Autodesk Inventor part; units mm, degrees
ref_plane "YZ Plane" through (0, 0, 0) normal (1, 0, 0) x (0, 1, 0)
ref_plane "XZ Plane" through (0, 0, 0) normal (0, 1, 0) x (-1, 0, 0)
ref_plane "XY Plane" through (0, 0, 0) normal (0, 0, 1) x (1, 0, 0)
sketch "Sketch1" plane through (0, 0, 0) normal (0, 0, 1) x (1, 0, 0)
  circle A0 centre (0, 0) radius 2.5
  dimension "d0" = 5
extrude "Extrusion1" add sketch "Sketch1" along normal blind 105
sketch "Sketch2" plane through (0, 0, 105) normal (0, 0, 1) x (1, 0, 0)
  circle A0 centre (0, 0) radius 2.5
  circle A1 centre (0, 0) radius 2.5
  circle A2 centre (0, 0) radius 3.75
  dimension "d3" = 7.5
extrude "Extrusion2" add sketch "Sketch2" against normal blind 105
fillet "Fillet1" radius 3 1 edges at (-3.75, 0, 105)
properties part number "Line"
CAD build for the part. Positions are in the model's coordinates, mm. Coordinates: 2 decimals unless noted, no trailing zeros. Order: outer loops, then holes, each group sorted by start corner. A loop starts at its lowest first (then second) coordinate and runs counter-clockwise, first axis right, second up. Notation, with made-up numbers: (65, -24.5) - (72, -24.5) arc R19 ccw to (72, -0.5) - close; hole circle Ø6 at (86, 12.5). An arc over 180 degrees is marked (long way). Answer in a Markdown table with one row per item.
1. Flat gauge pin, fed straight in: P1, Ø3, axis at y = 2, z = 70, coming from the -X side. Where does the tip first touch, or does it go through?
Answer:
| item | result |
|---|---|
| P1 | x = -3.72 |
2. Drill centre lines: L1, parallel to X at y = 0.25, z = 76; L2, parallel to X at y = -2.25, z = 70; L3, parallel to Z at x = -1.5, y = -0.5. Where is each one in solid material? Low to high. Write a range as from..to.
Answer:
| item | result |
|---|---|
| L1 | -3.74..3.74 |
| L2 | -3..3 |
| L3 | 0..104.88 |
3. Slice it at A-A, the plane z = 17.5. List the corners of the cut face in (x, y), then the cut area to 3 significant figures.
Answer:
| item | result |
|---|---|
| outline | circle Ø7.5 at (0, 0) |
| area | 44.2 mm² |
